Build history of the part. All positions in model axes, mm. A direction names the side the tool comes from. Give positions to 0.01 mm unless a question says otherwise; leave off trailing zeros. Order: outer loops, then holes, each group sorted by start corner. A loop starts at its lowest first (then second) coordinate and runs counter-clockwise, first axis right, second up. Notation, with made-up numbers: M 34,29 L 67,29 A15 cw 67,37 Z; hole C 89,45.25 d10. An arc over 180 degrees is marked long. One line per item, written item: value.
from build123d import *

# Parameters (mm, degrees)
F2_DEPTH = 3


with BuildPart() as f2:
    # F1 (on Top) → F2 (new body)
    with BuildSketch(Plane.XY):
        Polygon((10.5, -41), (10.5, -38), (29.5, -38), (29.5, -41), (53.5, -41), (53.5, -22), (50.5, -22), (50.5, -8), (53.5, -8), (53.5, 0), (53.5, 8), (50.5, 8), (50.5, 22), (53.5, 22), (53.5, 41), (29.5, 41), (29.5, 38), (10.5, 38), (10.5, 41), (0, 41), (-10.5, 41), (-10.5, 38), (-29.5, 38), (-29.5, 41), (-53.5, 41), (-53.5, 22), (-50.5, 22), (-50.5, 8), (-53.5, 8), (-53.5, 0), (-53.5, -8), (-50.5, -8), (-50.5, -22), (-53.5, -22), (-53.5, -41), (-29.5, -41), (-29.5, -38), (-10.5, -38), (-10.5, -41), (0, -41), align=None)
    extrude(amount=F2_DEPTH)


solid = f2.part
1) Saw through at A-A, the plane x = 15.5. Write the cut outline in (y, z).
Check values:
outline: M -38,0 L 38,0 L 38,3 L -38,3 Z
2) Pin check, flat tips, straight feed: pin 1 (1.5 mm diameter, centred on x = -18.5, z = 2, fed in from +Y); pin 2 (1.5 mm diameter, centred on y = -14, z = 1, fed in from +X). Stop position of each tip, or through.
Check values:
pin 1: y = 38
pin 2: x = 50.5
3) Tool access for faces 4 (the face through (52, 22, 1)), 5 (the face through (-20, -38, 1)), 6 (the face through (-50.5, 15, 1)): list every direction of +Z, -Z, +X, -X, +Y, -Y with a clear straight run to the whole face (end or side of a thin tool).
Check values:
face 4: +Z, -Z, +X
face 5: +Z, -Z, -Y
face 6: +Z, -Z, -X
4) Drill centre lines: probe 1 along X at (y, z) = (-9, 0.6); probe 2 along Y at (x, z) = (16.5, 0.25). Where is each one in solid material? Low to high. Write a range as from..to.
Check values:
probe 1: -50.5..50.5
probe 2: -38..38
5) Mould opens along X. For faces 1 (the face through (53.5, 0, 1)), 2 (the face through (-52, -8, 1)), 3 (the face through (-20, 38, 1)) say: released by +X, released by -X, zero draft, split by the parting line, or undercut.
Check values:
face 1: released by +X
face 2: zero draft
face 3: undercut
